Can you work these out from the model? Positions are in its coordinate system, mm. A direction names the side the tool comes from. Coordinates: 2 decimals unless noted, no trailing zeros. Loops run counter-clockwise (first coordinate to the right, second up) from the corner with the lowest first, then second, coordinate; pieces in that order, holes last. Notation, with made-up numbers: (17, -24) -> (32, -24) arc R10 cw to (32, -15) -> close; hole circle Ø6 at (40.5, 68.5). An arc over 180 degrees is marked (long way). Use one line per item in the form item = value. Start each with the question number.
(1) On a 3-axis mill with a long thin cutter (end or side, diameter ignored), from which of +Z, -Z, +X, -X, +Y, -Y can I reach the whole of each face in a straight line? I mean faces 4 (the flat face through (-1, -97, 12.7)), 5 (the flat face through (81, 77, 0)), 6 (the flat face through (285.75, 0, 243)). Say none if no direction works.
(2) Imagine slicing it at D-D (y = -82.5). List the corners of the cut face in (x, z) for me, plus the area to 3 significant figures.
(3) I'm going to push flat-ended pins straight in: pin 1 (1 mm diameter, centred on x = 146.5, z = 163, fed in from -Y); pin 2 (1 mm diameter, centred on y = 1, z = 411, fed in from -X); pin 3 (1 mm diameter, centred on x = -195, z = 401, fed in from +Y). Where does each tip first touch, or does it pass through?
(4) Imagine slicing it at A-A (x = -179). List the corners of the cut face in (y, z) for me (3 decimals), plus the area to 3 significant figures.
(5) Thinking about a two-plate mould opening in Z: for faces 1 (the flat face through (-4, 25.4, 243)), 2 (the flat face through (-128.588, -1, 22)), 3 (the flat face through (-83, 77, 0)), which applies, released by +Z, released by -Z, zero draft, split by the parting line, or undercut?
(6) I need wall thicknesses on line 1 (Z direction, x = 212.5, y = -14) (3 decimals); line 2 (Z direction, x = -129.5, y = 23.5) (3 decimals); line 3 (Y direction, x = 24, z = 226). Which ranges of each line are inside material? Lowest first, please. Write a range as [from, to].
(7) Imagine slicing it at B-B (y = -42.5). List the corners of the cut face in (x, z) for me, plus the area to 3 significant figures.
```python
from build123d import *

# Parameters (mm, degrees)
F1_DEPTH = 12.7
F2_W     = 876.3
F2_H     = 101.6
F3_DEPTH = 25.4
F4_W     = 257.175
F4_H     = 187.325
F5_DEPTH = 19.05
F6_W     = 571.5
F6_H     = 50.8
F7_DEPTH = 428.625


with BuildPart() as f1:
    # F0 (on Top) → F1 (new body)
    with BuildSketch(Plane.XY):
        with BuildLine():
            Line((-146.05, -101.6), (146.05, -101.6))
            ThreePointArc((146.05, -101.6), (150.540128, -99.740128), (152.4, -95.25))
            Line((152.4, -95.25), (152.4, 95.25))
            ThreePointArc((152.4, 95.25), (150.540128, 99.740128), (146.05, 101.6))
            Line((146.05, 101.6), (19.05, 101.6))
            ThreePointArc((19.05, 101.6), (14.559872, 99.740128), (12.7, 95.25))
            Line((12.7, 95.25), (12.7, 57.15))
            ThreePointArc((12.7, 57.15), (0, 44.45), (-12.7, 57.15))
            Line((-12.7, 57.15), (-12.7, 95.25))
            ThreePointArc((-12.7, 95.25), (-14.559872, 99.740128), (-19.05, 101.6))
            Line((-19.05, 101.6), (-146.05, 101.6))
            ThreePointArc((-146.05, 101.6), (-150.540128, 99.740128), (-152.4, 95.25))
            Line((-152.4, 95.25), (-152.4, -95.25))
            ThreePointArc((-152.4, -95.25), (-150.540128, -99.740128), (-146.05, -101.6))
        make_face()
    extrude(amount=F1_DEPTH)

    # F2 (on face) → F3 (join)
    with BuildSketch(Plane(origin=(0, 0, 0), x_dir=(1, 0, 0), z_dir=(0, 0, -1))):
        Rectangle(F2_W, F2_H)
    extrude(amount=F3_DEPTH)

    # F4 (on face) → F5 (join)
    with BuildSketch(Plane.XY.offset(12.7)):
        Rectangle(F4_W, F4_H)
    extrude(amount=F5_DEPTH)

    # F6 (on face) → F7 (join)
    with BuildSketch(Plane.XY.offset(31.75)):
        Rectangle(F6_W, F6_H)
    extrude(amount=F7_DEPTH)


solid = f1.part
```
Worked out:
q1.face_4 = none
q1.face_5 = -Z, +X, -X, +Y
q1.face_6 = +Z, +X, +Y, -Y
q2.outline = (-152.4, 0) -> (152.4, 0) -> (152.4, 12.7) -> (128.59, 12.7) -> (128.59, 31.75) -> (-128.59, 31.75) -> (-128.59, 12.7) -> (-152.4, 12.7) -> close
q2.area = 8,770 mm2
q3.pin_1 = -25.4
q3.pin_2 = -285.75
q3.pin_3 = 25.4
q4.outline = (-50.8, -25.4) -> (50.8, -25.4) -> (50.8, 0) -> (-50.8, 0) -> close; (-25.4, 31.75) -> (25.4, 31.75) -> (25.4, 460.375) -> (-25.4, 460.375) -> close
q4.area = 24,400 mm2
q5.face_1 = zero draft
q5.face_2 = undercut
q5.face_3 = released by -Z
q6.line_1 = [-25.4, 0], [31.75, 460.375]
q6.line_2 = [-25.4, 12.7], [31.75, 460.375]
q6.line_3 = [-25.4, 25.4]
q7.outline = (-438.15, -25.4) -> (438.15, -25.4) -> (438.15, 0) -> (152.4, 0) -> (152.4, 12.7) -> (128.59, 12.7) -> (128.59, 31.75) -> (-128.59, 31.75) -> (-128.59, 12.7) -> (-152.4, 12.7) -> (-152.4, 0) -> (-438.15, 0) -> close
q7.area = 31,000 mm2
